The model under review builds one solid part; all positions refer to its coordinate system, in mm. A direction names the side the tool comes from. Give positions to 0.01 mm unless a question says otherwise; leave off trailing zeros. Order: outer loops, then holes, each group sorted by start corner. A loop starts at its lowest first (then second) coordinate and runs counter-clockwise, first axis right, second up. Notation, with made-up numbers: (83, -38.75) - (96, -38.75) arc R11 ccw to (96, -31.75) - close; hole circle Ø2 at (53, -34). An arc over 180 degrees is marked (long way). Write item = value, one per line. Start each with the question number.
1. Mouldability with a two-part tool opening along Y and no side actions: class faces 4 (the cylindrical face through (-81, 3, 158)), 5 (the flat face through (-1, 3, 17)), 6 (the flat face through (-1, -3, 97)), 7 (the cylindrical face through (82, -4, 157)) as pulls with the +Y half, pulls with the -Y half, needs draft (parallel to the pull), parting line crosses it, or undercut.
2. Wall thickness on probe 1 along Z at (x, y) = (-67, -0.75); probe 2 along Z at (x, y) = (-25, -3.25); probe 3 along X at (y, z) = (-0.5, 160): over which ranges is each line inside the solid? List them lowest first.
3. Machinability: for faces 1 (the cylindrical face through (-82, -4, 158)), 2 (the flat face through (-1, 0, 30)), 3 (the flat face through (-80, 0, 24)), which of the approach directions +Z, -Z, +X, -X, +Y, -Y give a long, thin tool a straight path to every point of the face, cutting with its end or side? Answer none if there is none.
4. For P1, Ø1, axis at x = 15, y = -2.5, coming from the -Z side; P2, Ø12, axis at x = 53.5, z = 169.5, coming from the -Y side, all flat-tipped, find the tip position at first contact; note any pin that passes through.
5. We need section B-B, the plane z = 105.5. Give the boundary of the cut face in (x, y), and give its area (3 significant figures).
6. We need section A-A, the plane x = -71.5. State how many separate pieces and enclosed holes the cut face has, and give its area (3 significant figures).
from build123d import *

# Parameters (mm, degrees)
F0_W          = 160
F0_H          = 10
F0_H_2        = 40
F1_DEPTH      = 5
F1_DEPTH_BACK = 5
F2_F1_R       = 5
F2_F2_R       = 4.9999
F3_R          = 20
F4_W          = 160
F4_H          = 6
F5_DEPTH      = 6
F6_W          = 160
F6_H          = 6
F7_DEPTH      = 6


# Not quite as in the source:
# - a fillet or chamfer is up to 0.001 mm smaller than in the source, because OpenCascade refuses the exact size


with BuildPart() as f1:
    # F0 (on Front) → F1 (new body, two sides)
    with BuildSketch(Plane.XZ) as f1_sk:
        Polygon((-100, 0), (0, 0), (100, 0), (100, 200), (0, 200), (-100, 200), align=None)
        with Locations((0, 25)):
            Rectangle(F0_W, F0_H, mode=Mode.SUBTRACT)
        with Locations((0, 105)):
            Rectangle(F0_W, F0_H, mode=Mode.SUBTRACT)
        with Locations((0, 160)):
            Rectangle(F0_W, F0_H_2, mode=Mode.SUBTRACT)
    extrude(amount=F1_DEPTH)
    extrude(f1_sk.sketch, amount=-F1_DEPTH_BACK)

    # F2: fillet of radius 5 on 4 edges, made by hand

    # F2_f1
    f2_f1_edges = [f1.edges().sort_by_distance(p)[0] for p in [
        (80, 0, 180),
        (-80, 0, 180),
    ]]
    fillet(f2_f1_edges, radius=F2_F1_R)

    # F2_f2 (radius 5 in the source; OpenCascade refuses exactly that, so slightly less here)
    f2_f2_edges = [f1.edges().sort_by_distance(p)[0] for p in [
        (0, -5, 180),
        (0, 5, 180),
        (-78.5355339059, 5, 178.5355339059),
        (78.5355339059, 5, 178.5355339059),
        (-78.5355339059, -5, 178.5355339059),
        (78.5355339059, -5, 178.5355339059),
    ]]
    fillet(f2_f2_edges, radius=F2_F2_R)

    # F3
    f3_edges = [f1.edges().sort_by_distance(p)[0] for p in [
        (-100, 0, 200),
        (100, 0, 200),
    ]]
    fillet(f3_edges, radius=F3_R)

    # F4 (on face) → F5 (cut)
    with BuildSketch(Plane.XY.offset(20)):
        Rectangle(F4_W, F4_H)
    extrude(amount=-F5_DEPTH, mode=Mode.SUBTRACT)

    # F6 (on face) → F7 (cut)
    with BuildSketch(Plane.XY.offset(100)):
        Rectangle(F6_W, F6_H)
    extrude(amount=-F7_DEPTH, mode=Mode.SUBTRACT)


solid = f1.part
Model answer:
q1.face_4 = pulls with the +Y half
q1.face_5 = undercut
q1.face_6 = undercut
q1.face_7 = pulls with the -Y half
q2.probe_1 = 0 to 14, 30 to 94, 110 to 140, 180.06 to 200
q2.probe_2 = 0 to 20, 30 to 100, 110 to 140, 181.2 to 200
q2.probe_3 = -100 to -80.03, 80.03 to 100
q3.face_1 = -Y
q3.face_2 = +Y, -Y
q3.face_3 = none
q4.P1 = 0
q4.P2 = through
q5.outline = (-100, -5) - (-80, -5) - (-80, 5) - (-100, 5) - close; (80, -5) - (100, -5) - (100, 5) - (80, 5) - close
q5.area = 400 mm2
q6.separate_pieces = 4
q6.enclosed_holes = 0
q6.area = 1,320 mm2
